Read the model definition and answer for the solid it produces. Units are mm, in the model's axes. Round coordinates to 2 decimals unless told otherwise and drop trailing zeros. Order: outer loops, then holes, each group sorted by start corner. A loop starts at its lowest first (then second) coordinate and runs counter-clockwise, first axis right, second up. Notation, with made-up numbers: (26.5, 47.25) - (61.5, 47.25) arc R11 cw to (61.5, 65.25) - close; hole circle Ø9 at (17, 71.5). An arc over 180 degrees is marked (long way). Put each result on its own line as item: value. Start each with the question number.
Q1. Section A-A on x = 26.5 is taken. Give the vertices of the cut face in (y, z).
Q2. Each of these flat-tipped pins is pushed along its axis until it touches: pin 1 Ø5 at (x, y) = (-73.05, -41.75) entering from +Z; pin 2 Ø1 at (x, z) = (4, 0.5) entering from -Y; pin 3 Ø1.5 at (y, z) = (-31, 1) entering from +X. Where does it stop, or does it pass through?
Q3. Section B-B on y = -24 is taken. Give the vertices of the cut face in (x, z), then the cut area to 3 significant figures.
Q4. Section C-C on z = 1.1 is taken. Give the vertices of the cut face in (x, y), then the cut area to 3 significant figures.
Q5. Find the intervals of material crossed by line 1 along X through (y, z) = (-3.5, 3.1); line 2 along X through (y, z) = (-13.5, 0.85); line 3 along Y through (x, z) = (-50, 3.75), in increasing order. Write a range as from..to.
from build123d import *

# Parameters (mm, degrees)
SKETCH_1_W          = 150
SKETCH_1_H          = 42
EXTRUDE_1_DEPTH     = 2
SKETCH_2_R          = 1
CUT_EXTRUDE_1_DEPTH = 2
SKETCH_3_W          = 154
SKETCH_3_H          = 46
EXTRUDE_2_DEPTH     = 3
FILLET_2_R          = 6
FILLET_3_R          = 6
CUT_EXTRUDE_START   = 2
SKETCH_2_2_R        = 1
CUT_EXTRUDE_2_DEPTH = 2
SKETCH_4_R          = 2
CUT_EXTRUDE_3_DEPTH = 2


with BuildPart() as part:
    # 草图1 → 凸台-拉伸1 (new body)
    with BuildSketch(Plane.XY):
        with Locations((0.451807229, -22.248953788)):
            Rectangle(SKETCH_1_W, SKETCH_1_H)
    extrude(amount=EXTRUDE_1_DEPTH)

    # 草图2 → 切除-拉伸1 (cut)
    with BuildSketch(Plane.XY.offset(2)):
        with Locations((73.951807229, -41.748953788)):
            Circle(SKETCH_2_R)
        with Locations(Location((73.951807229, -2.748953788, 0), (0, 0, 180))):
            Circle(SKETCH_2_R)
        with Locations(Location((-73.048192771, -41.748953788, 0), (0, 0, 180))):
            Circle(SKETCH_2_R)
        with Locations((-73.048192771, -2.748953788)):
            Circle(SKETCH_2_R)
    extrude(amount=-CUT_EXTRUDE_1_DEPTH, mode=Mode.SUBTRACT)

    # 草图3 → 凸台-拉伸2 (add)
    with BuildSketch(Plane.XY.offset(2)):
        with Locations((0.451807229, -22.248953788)):
            Rectangle(SKETCH_3_W, SKETCH_3_H)
    extrude(amount=EXTRUDE_2_DEPTH)

    # 圆角2
    fillet_2_edges = [part.edges().sort_by_distance(p)[0] for p in [
        (-76.548192771, 0.751046212, 3.5),
        (-76.548192771, -45.248953788, 3.5),
        (77.451807229, -45.248953788, 3.5),
        (77.451807229, 0.751046212, 3.5),
    ]]
    fillet(fillet_2_edges, radius=FILLET_2_R)

    # 圆角3
    # the kernel refuses this fillet: 6 mm, written as the material it takes off along each edge
    with BuildSketch(Plane(origin=(71.451807229, -5.248953788, 5), x_dir=(0, 1, 0), z_dir=(-1, 0, 0))) as fillet_3_piece_1:
        with BuildLine():
            CenterArc((0.803847577, 6), FILLET_3_R, 270, 60)
            Line((0.803847577, 0), (0.803847577, -0.12))
            Line((0.803847577, -0.12), (6, -0.12))
            Line((6, -0.12), (6.12, 0))
            ThreePointArc((6.12, 0), (6.12, 1.5), (6.103923048, 2.94))
            Line((6.103923048, 2.94), (6, 3))
        make_face()
    revolve(axis=Axis((71.451807229, -5.248953788, 5), (0, 0, -1)), revolution_arc=90, mode=Mode.SUBTRACT)
    with BuildSketch(Plane(origin=(77.451807229, -5.248953788, 5), x_dir=(-1, 0, 0), z_dir=(0, -1, 0)), Plane(origin=(-76.548192771, -39.248953788, 5), x_dir=(1, 0, 0), z_dir=(0, 1, 0))) as fillet_3_piece_2:
        with BuildLine():
            CenterArc((5.196152423, 6), FILLET_3_R, 210, 60)
            Line((0, 3), (-0.103923048, 2.94))
            ThreePointArc((-0.103923048, 2.94), (-0.12, 1.5), (-0.12, 0))
            Line((-0.12, 0), (0, -0.12))
            Line((0, -0.12), (5.196152423, -0.12))
            Line((5.196152423, -0.12), (5.196152423, 0))
        make_face()
    extrude(amount=34, mode=Mode.SUBTRACT)
    with BuildSketch(Plane(origin=(71.451807229, -39.248953788, 5), x_dir=(1, 0, 0), z_dir=(0, 1, 0))) as fillet_3_piece_3:
        with BuildLine():
            CenterArc((0.803847577, 6), FILLET_3_R, 270, 60)
            Line((6, 3), (6.103923048, 2.94))
            ThreePointArc((6.103923048, 2.94), (6.12, 1.5), (6.12, 0))
            Line((6.12, 0), (6, -0.12))
            Line((6, -0.12), (0.803847577, -0.12))
            Line((0.803847577, -0.12), (0.803847577, 0))
        make_face()
    revolve(axis=Axis((71.451807229, -39.248953788, 5), (0, 0, -1)), revolution_arc=90, mode=Mode.SUBTRACT)
    with BuildSketch(Plane(origin=(71.451807229, -45.248953788, 5), x_dir=(0, 1, 0), z_dir=(-1, 0, 0))) as fillet_3_piece_4:
        with BuildLine():
            CenterArc((5.196152423, 6), FILLET_3_R, 210, 60)
            Line((0, 3), (-0.103923048, 2.94))
            ThreePointArc((-0.103923048, 2.94), (-0.12, 1.5), (-0.12, 0))
            Line((-0.12, 0), (0, -0.12))
            Line((0, -0.12), (5.196152423, -0.12))
            Line((5.196152423, -0.12), (5.196152423, 0))
        make_face()
    extrude(amount=142, mode=Mode.SUBTRACT)
    with BuildSketch(Plane(origin=(-70.548192771, -39.248953788, 5), x_dir=(-1, 0, 0), z_dir=(0, 1, 0))) as fillet_3_piece_5:
        with BuildLine():
            CenterArc((0.803847577, -6), FILLET_3_R, 30, 60)
            Line((6, -3), (6.103923048, -2.94))
            ThreePointArc((6.103923048, -2.94), (6.12, -1.5), (6.12, 0))
            Line((6.12, 0), (6, 0.12))
            Line((6, 0.12), (0.803847577, 0.12))
            Line((0.803847577, 0.12), (0.803847577, 0))
        make_face()
    revolve(axis=Axis((-70.548192771, -39.248953788, 5), (0, 0, 1)), revolution_arc=90, mode=Mode.SUBTRACT)
    with BuildSketch(Plane(origin=(-70.548192771, -5.248953788, 5), x_dir=(0, 1, 0), z_dir=(1, 0, 0))) as fillet_3_piece_6:
        with BuildLine():
            CenterArc((0.803847577, -6), FILLET_3_R, 30, 60)
            Line((0.803847577, 0), (0.803847577, 0.12))
            Line((0.803847577, 0.12), (6, 0.12))
            Line((6, 0.12), (6.12, 0))
            ThreePointArc((6.12, 0), (6.12, -1.5), (6.103923048, -2.94))
            Line((6.103923048, -2.94), (6, -3))
        make_face()
    revolve(axis=Axis((-70.548192771, -5.248953788, 5), (0, 0, 1)), revolution_arc=90, mode=Mode.SUBTRACT)
    with BuildSketch(Plane(origin=(-70.548192771, 0.751046212, 5), x_dir=(0, 0, -1), z_dir=(1, 0, 0))) as fillet_3_piece_7:
        with BuildLine():
            CenterArc((6, -5.196152423), FILLET_3_R, 120, 60)
            Line((0, -5.196152423), (-0.12, -5.196152423))
            Line((-0.12, -5.196152423), (-0.12, 0))
            Line((-0.12, 0), (0, 0.12))
            ThreePointArc((0, 0.12), (1.5, 0.12), (2.94, 0.103923048))
            Line((2.94, 0.103923048), (3, 0))
        make_face()
    extrude(amount=142, mode=Mode.SUBTRACT)

    # 草图2<2> → 切除-拉伸2 (cut)
    with BuildSketch(Plane.XY.offset(2).offset(CUT_EXTRUDE_START)):
        with Locations((73.951807229, -41.748953788)):
            Circle(SKETCH_2_2_R)
        with Locations(Location((73.951807229, -2.748953788, 0), (0, 0, 344.465859099))):
            Circle(SKETCH_2_2_R)
        with Locations(Location((-73.048192771, -41.748953788, 0), (0, 0, 285.534141265))):
            Circle(SKETCH_2_2_R)
        with Locations((-73.048192771, -2.748953788)):
            Circle(SKETCH_2_2_R)
    extrude(amount=-CUT_EXTRUDE_2_DEPTH, mode=Mode.SUBTRACT)

    # 草图4 → 切除-拉伸3 (cut)
    with BuildSketch(Plane.XY.offset(5)):
        with Locations((73.951807229, -2.748953788)):
            Circle(SKETCH_4_R)
        with Locations((73.951807229, -41.748953788)):
            Circle(SKETCH_4_R)
        with Locations((-73.048192771, -41.748953788)):
            Circle(SKETCH_4_R)
        with Locations((-73.048192771, -2.748953788)):
            Circle(SKETCH_4_R)
    extrude(amount=-CUT_EXTRUDE_3_DEPTH, mode=Mode.SUBTRACT)


solid = part.part
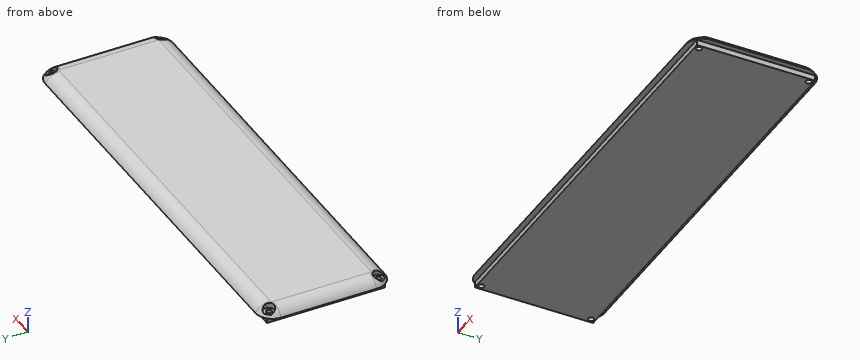
Findings:
1. outline: (-45.25, 2) - (-43.25, 2) - (-43.25, 0) - (-1.25, 0) - (-1.25, 2) - (0.75, 2) arc R6 ccw to (-4.45, 5) - (-40.05, 5) arc R6 ccw to start
2. pin 1: z = 5
2. pin 2: y = -43.25
2. pin 3: x = 75.45
3. outline: (-76.55, 2) - (-74.55, 2) - (-74.55, 0) - (75.45, 0) - (75.45, 2) - (77.45, 2) arc R6 ccw to (72.26, 5) - (-71.35, 5) arc R6 ccw to start
3. area: 753 mm2
4. outline: (-74.55, -43.25) - (75.45, -43.25) - (75.45, -1.25) - (-74.55, -1.25) - close; hole circle Ø2 at (-73.05, -41.75); hole circle Ø2 at (-73.05, -2.75); hole circle Ø2 at (73.95, -41.75); hole circle Ø2 at (73.95, -2.75)
4. area: 6,290 mm2
5. line 1: -75.43..-74.9, -71.19..72.1, 75.81..76.33
5. line 2: -74.55..75.45
5. line 3: -43.72..-0.78
